Autodesk Inventor part; units mm, degrees
ref_plane "YZ Plane" through (0, 0, 0) normal (1, 0, 0) x (0, 1, 0)
ref_plane "XZ Plane" through (0, 0, 0) normal (0, 1, 0) x (-1, 0, 0)
ref_plane "XY Plane" through (0, 0, 0) normal (0, 0, 1) x (1, 0, 0)
sketch "Sketch4" plane through (0, 0, 0) normal (0, 1, 0) x (-1, 0, 0)
  line L0 (-102.6818, 131.0909) -> (-102.6818, 58.0909) construction
  line L1 (24.8182, 125) -> (-230.1818, 125)
  line L2 (-230.1818, 125) -> (-230.1818, 135)
  line L3 (-230.1818, 135) -> (24.8182, 135)
  line L4 (24.8182, 135) -> (24.8182, 125)
  line L5 (24.8182, 125) -> (-230.1818, 135) construction
  line L6 (-230.1818, 125) -> (24.8182, 135) construction
  line L7 (0, 0) -> (36.133, 0) construction
  line L8 (24.8182, -125) -> (-230.1818, -125)
  line L9 (-230.1818, -125) -> (-230.1818, -135)
  line L10 (-230.1818, -135) -> (24.8182, -135)
  line L11 (24.8182, -135) -> (24.8182, -125)
  line L12 (24.8182, -125) -> (-230.1818, -135) construction
  line L13 (-230.1818, -125) -> (24.8182, -135) construction
  point P0 (-102.6818, 130)
  dimension "d4" = 10
  dimension "d6" = 250
  dimension "d7" = 255
extrude "Extrusion2" add sketch "Sketch4" along normal blind 10
sketch "Sketch9" plane through (230.1818, 0, -125) normal (1, 0, 0) x (0, 0, -1)
  line L0 (-125, 0) -> (-125, -106.9842) construction
  line L1 (10, 0) -> (10, 10) construction
  line L2 (0, 10) -> (10, 10) construction
  line L3 (10, 0) -> (0, 10) construction
  line L4 (0, 10) -> (10, 10) construction
  line L5 (10, 10) -> (0, 0) construction
  circle A0 centre (5, 5) radius 5
  line L6 (-260, 0) -> (-260, 10) construction
  line L7 (-250, 10) -> (-260, 10) construction
  line L8 (-260, 0) -> (-250, 10) construction
  line L9 (-250, 10) -> (-260, 10) construction
  line L10 (-260, 10) -> (-250, 0) construction
  circle A1 centre (-255, 5) radius 5
extrude "Extrusion3" cut sketch "Sketch9" against normal through all keep common part
sketch "Sketch10" plane through (230.1818, 5, -130) normal (1, 0, 0) x (0, 0, -1)
  circle A0 centre (0, 0) radius 5 construction
  line L0 (0, 5) -> (-260, 5)
  line L1 (-130, -5) -> (-130, 5) construction
  line L2 (-155, -155.4301) -> (-105, -155.4301)
  line L3 (-105, -155.4301) -> (-105, -145)
  line L4 (-105, -145) -> (-155, -145)
  line L5 (-155, -145) -> (-155, -155.4301)
  line L6 (-155, -155.4301) -> (-105, -145) construction
  line L7 (-105, -155.4301) -> (-155, -145) construction
  line L8 (-130, -150.215) -> (-130, -124.8826) construction
  dimension "d13" = 150
  dimension "d34" = 50
extrude "Extrusion4" add sketch "Sketch10" against normal blind 255
sketch "Sketch11" plane through (230.1818, 5, -130) normal (1, 0, 0) x (0, 0, -1)
  circle A0 centre (0, 0) radius 5
  line L0 (-155, -145) -> (-105, -145)
  line L1 (-130, 0) -> (-130, -145) construction
  line L2 (-130, -145) -> (-286.0792, -145) construction
  line L3 (-130, -145) -> (0, -145) construction
  circle A1 centre (-60, -145) radius 5
  circle A2 centre (-200, -145) radius 5
  line L4 (-55, -145) -> (4.6154, -1.9231)
  circle A3 centre (-260, 0) radius 5
  line L5 (-190, -245.9934) -> (-70, -245.9934)
  line L6 (-70, -245.9934) -> (-70, -195.9934)
  line L7 (-70, -195.9934) -> (-190, -195.9934)
  line L8 (-190, -195.9934) -> (-190, -245.9934)
  line L9 (-190, -245.9934) -> (-70, -195.9934) construction
  line L10 (-70, -245.9934) -> (-190, -195.9934) construction
  line L11 (-130, -220.9934) -> (-130, -179.9046) construction
  line L12 (-55, -145) -> (-76.2472, -195.9934)
  line L13 (-5, 0) -> (-65, -145)
  line L14 (-65, -145) -> (-86.1007, -195.9934)
  line L15 (-255, 0) -> (-195, -145)
  line L16 (-263.5381, -3.533) -> (-205, -145)
  line L17 (-195, -145) -> (-173.8993, -195.9934)
  line L18 (-205, -145) -> (-183.8993, -195.9934)
  point P0 (-130, -5)
  dimension "d18" = 10
  dimension "d20" = 140
  dimension "d21" = 120
  dimension "d22" = 50
extrude "Extrusion5" add sketch "Sketch11" against normal blind 255 contours A0 L4 A1 L13 | A1 L12 L13 | A1 L12 L7 L14 | L7 L6 L5 L8 | L7 L18 A2 L17 | A2 L18 L15 | A2 L16 A3 L15
sketch "Sketch12" plane through (-24.8182, 5, -130) normal (-1, 0, 0) x (0, 0, 1)
  line L0 (173.8993, -195.9934) -> (86.1007, -195.9934)
  line L1 (105, -155.4301) -> (155, -155.4301)
  line L2 (86.1007, -195.9934) -> (173.8993, -195.9934)
  line L3 (152.374, -195.9934) -> (149.1071, -155.4301)
  line L4 (142.3416, -195.9934) -> (139.0748, -155.4301)
  line L5 (155, -155.4301) -> (105, -155.4301)
  line L6 (255, 0) -> (173.8993, -195.9934)
  line L7 (86.1007, -195.9934) -> (5, 0)
  line L8 (173.8993, -195.9934) -> (105, -155.4301) construction
  line L9 (155, -155.4301) -> (86.1007, -195.9934) construction
  line L10 (130, -170.1484) -> (130, -155.4301) construction
  line L11 (107.626, -195.9934) -> (110.8929, -155.4301)
  line L12 (117.6584, -195.9934) -> (120.9252, -155.4301)
  point P0 (130, -5)
  point P1 (107.626, -195.9934)
  point P2 (117.6584, -195.9934)
  dimension "d25" = 10
extrude "Extrusion6" add sketch "Sketch12" against normal blind 255 contours L0 L4 L1 L3 | L0 L11 L1 L12
sketch "Sketch13" plane through (230.1818, -240.9934, -60) normal (0, 0, -1) x (-1, 0, 0)
  line L0 (0, 50) -> (255, 50)
  line L1 (0, 50) -> (0, 244.0703)
  line L2 (0, 50) -> (255, 50)
  line L3 (255, 244.0703) -> (255, 50)
  line L4 (0, 244.0703) -> (255, 244.0703)
  line L5 (0, 90.5633) -> (255, 90.5633)
  line L6 (0, 100.9934) -> (255, 100.9934)
  line L7 (0, 0) -> (255, 0)
  line L8 (0, 0) -> (0, 50)
  line L9 (255, 50) -> (255, 0)
  line L10 (255, 100.9934) -> (0, 244.0703) construction
  line L11 (1.2728, 100.9934) -> (255, 244.0703) construction
  line L12 (138.1364, 100.9934) -> (118.1364, 100.9934)
  line L13 (118.1364, 100.9934) -> (118.1364, 244.0703)
  line L14 (118.1364, 244.0703) -> (138.1364, 244.0703)
  line L15 (138.1364, 244.0703) -> (138.1364, 100.9934)
  line L16 (138.1364, 100.9934) -> (118.1364, 244.0703) construction
  line L17 (118.1364, 100.9934) -> (138.1364, 244.0703) construction
  point P0 (230.1818, 240.9934)
  point P1 (128.1364, 172.5318)
  point P2 (138.1364, 100.9934)
  point P3 (118.1364, 100.9934)
  dimension "d28" = 20
extrude "Extrusion7" cut sketch "Sketch13" along normal mid plane 434.75 contours L1 L4 L13 L6 | L6 L15 L4 L3
sketch "Sketch14" plane through (230.1818, -240.9934, -60) normal (0, 0, -1) x (-1, 0, 0)
  line L0 (0, 50) -> (255, 50)
  line L1 (255, 100.9934) -> (255, 50)
  line L2 (255, 50) -> (255, 0)
  line L3 (255, 100.9934) -> (138.1364, 100.9934)
  line L4 (0, 0) -> (255, 0)
  line L5 (0, 0) -> (0, 50)
  line L6 (0, 90.5633) -> (255, 90.5633)
  line L7 (0, 100.9934) -> (118.1364, 100.9934)
  line L8 (0, 100.9934) -> (0, 50)
  line L9 (118.1364, 100.9934) -> (138.1364, 100.9934)
  line L10 (128.1364, 88.0174) -> (128.1364, 65.5782) construction
  line L11 (255, 90.5633) -> (0, 100.9934) construction
  line L12 (0, 90.5633) -> (255, 100.9934) construction
  line L13 (127.5, 95.7783) -> (127.5, 90.5633) construction
  line L14 (0, 50) -> (255, 50)
  line L15 (77.5, 50) -> (177.5, 50)
  line L16 (177.5, 50) -> (177.5, 100.9934)
  line L17 (177.5, 100.9934) -> (77.5, 100.9934)
  line L18 (77.5, 100.9934) -> (77.5, 50)
  line L19 (177.5, 50) -> (77.5, 100.9934) construction
  line L20 (177.5, 100.9934) -> (77.5, 50) construction
  line L21 (127.5, 75.4967) -> (127.5, 84.9841) construction
  point P0 (230.1818, 240.9934)
  point P1 (77.5, 50)
  point P2 (77.5, 100.9934)
  point P3 (177.5, 100.9934)
  dimension "d31" = 100
extrude "Extrusion8" cut sketch "Sketch14" along normal mid plane 434.75 contours L8 L6 L18 L0 | L8 L7 L18 L6 | L16 L6 L1 L0 | L16 L3 L1 L6
properties part number "drone model"
Part model, mm, in its own coordinate system. A direction names the side the tool comes from. Coordinates: 2 decimals unless noted, no trailing zeros. Loops run counter-clockwise (first coordinate to the right, second up) from the corner with the lowest first, then second, coordinate; pieces in that order, holes last. Notation, with made-up numbers: (2, -8.75) -> (42, -8.75) arc R9 cw to (42, 4.25) -> close; hole circle Ø2 at (34.25, 82). An arc over 180 degrees is marked (long way). Use a Markdown table: item, result. Add a question column.
Item 1: Flat gauge pins, fed straight in: P1, Ø5, axis at x = 61, z = 65.5, coming from the +Y side; P2, Ø15, axis at x = 74.5, y = -206, coming from the -Z side; P3, Ø9.5, axis at y = -166.5, z = 54.5, coming from the -X side. Where does each tip first touch, or does it go through?
Item 2: Pull direction Y, two halves, no side cores. Call faces 6 (the flat face through (112.045, -69, 100)), 7 (the flat face through (103, -150.43, 0)), 8 (the flat face through (34, 3.077, -129)), 9 (the flat face through (101.982, -170.996, -20.763)): +Y half, -Y half, draft (parallel to the pull), parting line (faces both ways), or undercut.
Item 3: Which spindle directions (+Z, -Z, +X, -X, +Y, -Y) get a long thin tool onto all of the face, cutting with end or side? Do faces 1 (the flat face through (103, -145, 25)), 2 (the flat face through (34, 3.077, 129)), 3 (the flat face through (73, -140, -70)), 4 (the flat face through (152.682, -165, -59)), 5 (the flat face through (172, 3.077, 129)). Say none if no direction does.
Item 4: Band-saw the part on A-A on x = 123. Give the number of separate pieces and of enclosed holes in the cut face, plus the area to 3 significant figures.
Item 5: Band-saw the part on C-C on z = -130. Write the cut outline in (x, y), plus the area to 3 significant figures.
Item 6: Probe probe 1 along Y at (x, z) = (110.5, 2.5); probe 2 along Y at (x, z) = (156.5, -20.5); probe 3 along Z at (x, y) = (32, -194.5). List the from-to ranges inside material, lowest first.
Item 7: Band-saw the part on B-B on y = -40. Write the cut outline in (x, z).
Geometry says:
| question | item | result |
|---|---|---|
| 1 | P1 | y = -140 |
| 1 | P2 | z = -60 |
| 1 | P3 | x = 52.68 |
| 2 | face 6 | draft |
| 2 | face 7 | undercut |
| 2 | face 8 | -Y half |
| 2 | face 9 | undercut |
| 3 | face 1 | +X, -X, +Y |
| 3 | face 2 | +Z, -Z, -X, -Y |
| 3 | face 3 | +Z, -Z, -X, +Y |
| 3 | face 4 | +Z, -Z, +X, +Y |
| 3 | face 5 | +Z, -Z, +X, -Y |
| 4 | separate pieces | 3 |
| 4 | enclosed holes | 1 |
| 4 | area | 8,470 mm² |
| 5 | outline | (-24.82, 3.08) -> (92.05, 3.08) -> (92.05, -8) -> (112.05, -8) -> (112.05, 3.08) -> (230.18, 3.08) -> (230.18, 10) -> (-24.82, 10) -> close |
| 5 | area | 1,990 mm² |
| 6 | probe 1 | -240.99 to -190.99, -150.43 to -140 |
| 6 | probe 2 | -240.99 to -190.99 |
| 6 | probe 3 | -60 to 60 |
| 7 | outline | (92.05, -116.67) -> (112.05, -116.67) -> (112.05, -106.38) -> (92.05, -106.38) -> close; (92.05, 106.38) -> (112.05, 106.38) -> (112.05, 116.38) -> (92.05, 116.38) -> close |
